from build123d import *

# Parameters (mm, degrees)
F1_DEPTH = 50


with BuildPart() as f1:
    # F0 (on Front) → F1 (new body)
    with BuildSketch(Plane.XZ):
        with BuildLine():
            ThreePointArc((0, 1.5), (0.43934, 0.43934), (1.5, 0))
            Line((1.5, 0), (6.5, 0))
            Line((6.5, 0), (6.5, 0.5))
            Line((6.5, 0.5), (7, 0.5))
            Line((7, 0.5), (7, 1.5))
            Line((7, 1.5), (4, 1.5))
            Line((4, 1.5), (4, 3))
            Line((4, 3), (6.5, 5.5))
            Line((6.5, 5.5), (9.5, 5.5))
            Line((9.5, 5.5), (10, 5.75))
            Line((10, 5.75), (10.5, 5.5))
            Line((10.5, 5.5), (13.5, 5.5))
            Line((13.5, 5.5), (16, 3))
            Line((16, 3), (16, 1.5))
            Line((16, 1.5), (13, 1.5))
            Line((13, 1.5), (13, 0.5))
            Line((13, 0.5), (13.5, 0.5))
            Line((13.5, 0.5), (13.5, 0))
            Line((13.5, 0), (18.5, 0))
            ThreePointArc((18.5, 0), (19.56066, 0.43934), (20, 1.5))
            Line((20, 1.5), (20, 6.5))
            Line((20, 6.5), (19.5, 6.5))
            Line((19.5, 6.5), (19.5, 7))
            Line((19.5, 7), (18.5, 7))
            Line((18.5, 7), (18.5, 4))
            Line((18.5, 4), (17, 4))
            Line((17, 4), (14.5, 6.5))
            Line((14.5, 6.5), (14.5, 9.5))
            Line((14.5, 9.5), (14.25, 10))
            Line((14.25, 10), (14.5, 10.5))
            Line((14.5, 10.5), (14.5, 13.5))
            Line((14.5, 13.5), (17, 16))
            Line((17, 16), (18.5, 16))
            Line((18.5, 16), (18.5, 13))
            Line((18.5, 13), (19.5, 13))
            Line((19.5, 13), (19.5, 13.5))
            Line((19.5, 13.5), (20, 13.5))
            Line((20, 13.5), (20, 46.5))
            Line((20, 46.5), (19.5, 46.5))
            Line((19.5, 46.5), (19.5, 47))
            Line((19.5, 47), (18.5, 47))
            Line((18.5, 47), (18.5, 44))
            Line((18.5, 44), (17, 44))
            Line((17, 44), (14.5, 46.5))
            Line((14.5, 46.5), (14.5, 49.5))
            Line((14.5, 49.5), (14.25, 50))
            Line((14.25, 50), (14.5, 50.5))
            Line((14.5, 50.5), (14.5, 53.5))
            Line((14.5, 53.5), (17, 56))
            Line((17, 56), (18.5, 56))
            Line((18.5, 56), (18.5, 53))
            Line((18.5, 53), (19.5, 53))
            Line((19.5, 53), (19.5, 53.5))
            Line((19.5, 53.5), (20, 53.5))
            Line((20, 53.5), (20, 58.5))
            ThreePointArc((20, 58.5), (19.56066, 59.56066), (18.5, 60))
            Line((18.5, 60), (13.5, 60))
            Line((13.5, 60), (13.5, 59.5))
            Line((13.5, 59.5), (13, 59.5))
            Line((13, 59.5), (13, 58.5))
            Line((13, 58.5), (16, 58.5))
            Line((16, 58.5), (16, 57))
            Line((16, 57), (13.5, 54.5))
            Line((13.5, 54.5), (10.5, 54.5))
            Line((10.5, 54.5), (10, 54.25))
            Line((10, 54.25), (9.5, 54.5))
            Line((9.5, 54.5), (6.5, 54.5))
            Line((6.5, 54.5), (4, 57))
            Line((4, 57), (4, 58.5))
            Line((4, 58.5), (7, 58.5))
            Line((7, 58.5), (7, 59.5))
            Line((7, 59.5), (6.5, 59.5))
            Line((6.5, 59.5), (6.5, 60))
            Line((6.5, 60), (1.5, 60))
            ThreePointArc((1.5, 60), (0.43934, 59.56066), (0, 58.5))
            Line((0, 58.5), (0, 53.5))
            Line((0, 53.5), (0.5, 53.5))
            Line((0.5, 53.5), (0.5, 53))
            Line((0.5, 53), (1.5, 53))
            Line((1.5, 53), (1.5, 56))
            Line((1.5, 56), (3, 56))
            Line((3, 56), (5.5, 53.5))
            Line((5.5, 53.5), (5.5, 50.5))
            Line((5.5, 50.5), (5.75, 50))
            Line((5.75, 50), (5.5, 49.5))
            Line((5.5, 49.5), (5.5, 46.5))
            Line((5.5, 46.5), (3, 44))
            Line((3, 44), (1.5, 44))
            Line((1.5, 44), (1.5, 47))
            Line((1.5, 47), (0.5, 47))
            Line((0.5, 47), (0.5, 46.5))
            Line((0.5, 46.5), (0, 46.5))
            Line((0, 46.5), (0, 13.5))
            Line((0, 13.5), (0.5, 13.5))
            Line((0.5, 13.5), (0.5, 13))
            Line((0.5, 13), (1.5, 13))
            Line((1.5, 13), (1.5, 16))
            Line((1.5, 16), (3, 16))
            Line((3, 16), (5.5, 13.5))
            Line((5.5, 13.5), (5.5, 10.5))
            Line((5.5, 10.5), (5.75, 10))
            Line((5.75, 10), (5.5, 9.5))
            Line((5.5, 9.5), (5.5, 6.5))
            Line((5.5, 6.5), (3, 4))
            Line((3, 4), (1.5, 4))
            Line((1.5, 4), (1.5, 7))
            Line((1.5, 7), (0.5, 7))
            Line((0.5, 7), (0.5, 6.5))
            Line((0.5, 6.5), (0, 6.5))
            Line((0, 6.5), (0, 1.5))
        make_face()
        with BuildLine():
            Line((8.659501, 7.598841), (7.932254, 6.871594))
            ThreePointArc((7.932254, 6.871594), (7.34835, 7.34835), (6.871594, 7.932254))
            Line((6.871594, 7.932254), (7.598841, 8.659501))
            ThreePointArc((7.598841, 8.659501), (7.25, 10), (7.598841, 11.340499))
            Line((7.598841, 11.340499), (6.871594, 12.067746))
            ThreePointArc((6.871594, 12.067746), (7.34835, 12.65165), (7.932254, 13.128406))
            Line((7.932254, 13.128406), (8.659501, 12.401159))
            ThreePointArc((8.659501, 12.401159), (10, 12.75), (11.340499, 12.401159))
            Line((11.340499, 12.401159), (12.067746, 13.128406))
            ThreePointArc((12.067746, 13.128406), (12.65165, 12.65165), (13.128406, 12.067746))
            Line((13.128406, 12.067746), (12.401159, 11.340499))
            ThreePointArc((12.401159, 11.340499), (12.75, 10), (12.401159, 8.659501))
            Line((12.401159, 8.659501), (13.128406, 7.932254))
            ThreePointArc((13.128406, 7.932254), (12.65165, 7.34835), (12.067746, 6.871594))
            Line((12.067746, 6.871594), (11.340499, 7.598841))
            ThreePointArc((11.340499, 7.598841), (10, 7.25), (8.659501, 7.598841))
        make_face(mode=Mode.SUBTRACT)
        Polygon((1.5, 42.5), (3.62132, 42.5), (6.62132, 45.5), (10, 45.5), (13.37868, 45.5), (16.37868, 42.5), (18.5, 42.5), (18.5, 30), (18.5, 17.5), (16.37868, 17.5), (13.37868, 14.5), (10, 14.5), (6.62132, 14.5), (3.62132, 17.5), (1.5, 17.5), (1.5, 30), align=None, mode=Mode.SUBTRACT)
        with BuildLine():
            ThreePointArc((8.659501, 52.401159), (10, 52.75), (11.340499, 52.401159))
            Line((11.340499, 52.401159), (12.067746, 53.128406))
            ThreePointArc((12.067746, 53.128406), (12.65165, 52.65165), (13.128406, 52.067746))
            Line((13.128406, 52.067746), (12.401159, 51.340499))
            ThreePointArc((12.401159, 51.340499), (12.75, 50), (12.401159, 48.659501))
            Line((12.401159, 48.659501), (13.128406, 47.932254))
            ThreePointArc((13.128406, 47.932254), (12.65165, 47.34835), (12.067746, 46.871594))
            Line((12.067746, 46.871594), (11.340499, 47.598841))
            ThreePointArc((11.340499, 47.598841), (10, 47.25), (8.659501, 47.598841))
            Line((8.659501, 47.598841), (7.932254, 46.871594))
            ThreePointArc((7.932254, 46.871594), (7.34835, 47.34835), (6.871594, 47.932254))
            Line((6.871594, 47.932254), (7.598841, 48.659501))
            ThreePointArc((7.598841, 48.659501), (7.25, 50), (7.598841, 51.340499))
            Line((7.598841, 51.340499), (6.871594, 52.067746))
            ThreePointArc((6.871594, 52.067746), (7.34835, 52.65165), (7.932254, 53.128406))
            Line((7.932254, 53.128406), (8.659501, 52.401159))
        make_face(mode=Mode.SUBTRACT)
    extrude(amount=F1_DEPTH)


solid = f1.part
For this review, take the finished solid that the model builds, in its own axes (mm). Coordinates: 2 decimals unless noted, no trailing zeros. Order: outer loops, then holes, each group sorted by start corner. A loop starts at its lowest first (then second) coordinate and runs counter-clockwise, first axis right, second up. Notation, with made-up numbers: (20, 11) - (48, 11) arc R16 ccw to (48, 28) - close; hole circle Ø11 at (53, 83). An arc over 180 degrees is marked (long way). Use one line per item in the form item = value.
Q1. Consider section B-B (y = -6). Give the number of separate pieces and of enclosed holes in the cut face, then the cut area to 3 significant figures.
Checked values:
separate_pieces = 1
enclosed_holes = 3
area = 347 mm2
Q2. Consider section A-A (z = 30). Give the boundary of the cut face in (x, y), then the cut area to 3 significant figures.
Checked values:
outline = (0, -50) - (1.5, -50) - (1.5, 0) - (0, 0) - close; (18.5, -50) - (20, -50) - (20, 0) - (18.5, 0) - close
area = 150 mm2
Q3. For probe 1 along Z at (x, y) = (1.75, -24); probe 2 along X at (y, z) = (-13, 24.5); probe 3 along Z at (x, y) = (13.75, -23.5), list the stretches that pass through material, from the lowest coordinate up. Write a range as from..to.
Checked values:
probe_1 = 0..4, 16..17.5, 42.5..44, 56..60
probe_2 = 0..1.5, 18.5..20
probe_3 = 0..1.5, 5.25..14.87, 45.13..54.75, 58.5..60
Q4. For P1, Ø4, axis at x = 15, z = 25.5, coming from the +Y side; P2, Ø3.5, axis at y = -17.5, z = 11.5, coming from the +X side; P3, Ø0.5, axis at y = -16, z = 1, coming from the +X side, all flat-tipped, find the tip position at first contact; note any pin that passes through.
Checked values:
P1 = through
P2 = 19.5
P3 = 19.98
Q5. Draft analysis for pull direction Z (two halves, no side actions). For faces 1 (the flat face through (16, -25, 45)), 2 (the flat face through (1, 0, 30)), state which applies: +Z half, -Z half, draft (parallel to the pull), parting line (faces both ways), or undercut.
Checked values:
face_1 = undercut
face_2 = draft
